Source: CAD feature listing. Evaluate the final solid. Frame: model axes, mm. Face numbers are marked on the shaded views. A direction names the side the tool comes from. Round coordinates to 2 decimals unless told otherwise and drop trailing zeros. Write each loop counter-clockwise with the first axis right and the second up, starting at its lowest first coordinate (ties: lowest second). Pieces come first, ordered by that corner, then holes. Notation, with made-up numbers: (-5.5, 10.5) -> (19.5, 10.5) arc R16 ccw to (19.5, 22.5) -> close; hole circle Ø8 at (17.5, 58). An arc over 180 degrees is marked (long way). Put each result on its own line as item: value.
```python
from build123d import *

# Parameters (mm, degrees)
F1_DEPTH    = 76.2
F2_R        = 5.08
F3_T1_DEPTH = 76.2
F3_T4_ANGLE = 106.3398594687
F3_T6_ANGLE = 106.3398594687
F4_R        = 7.7543468395
F5_DEPTH    = 0.254
F6_DEPTH    = 5.08
F7_R        = 7.6382634684
F8_DEPTH    = 5.08
F10_R       = 7.2706121331
F11_DEPTH   = 5.08
F9_R        = 7.2450103535
F12_DEPTH   = 5.08
F13_R       = 2.3168995741
F14_DEPTH   = 10.16


# Not quite as in the source:
# - a fillet or chamfer that OpenCascade refuses, or shapes differently, is made with other operations: its cross-section is extruded or revolved along the edge and cut away or added
# - the program builds the solid bodies; features that only make, move or delete a surface that nothing else refers to are left out


with BuildPart() as f1:
    # F0 (on Front) → F1 (new body)
    with BuildSketch(Plane.XZ):
        Polygon((-120.808057487, 0), (-130.5492073298, -33.2263112068), (126.3735592365, -33.2263112068), (118.6618208885, 7.3618022725), (26.1209160089, 7.3618022725), (26.1209160089, 33.3381965756), (-76.9728943706, 33.3381965756), align=None)
    extrude(amount=F1_DEPTH)

    # F2
    f2_edges = [f1.edges().sort_by_distance(p)[0] for p in [
        (-125.678632, -76.2, -16.613156),
        (-98.890476, -76.2, 16.669098),
        (-25.425989, -76.2, 33.338197),
        (26.120916, -76.2, 20.349999),
        (26.120916, 0, 20.349999),
        (26.120916, -38.1, 33.338197),
        (-98.890476, 0, 16.669098),
        (-25.425989, 0, 33.338197),
        (-125.678632, 0, -16.613156),
        (-2.087824, 0, -33.226311),
        (-120.808057, -38.1, 0),
        (-2.087824, -76.2, -33.226311),
        (72.391368, -76.2, 7.361802),
        (118.661821, -38.1, 7.361802),
        (122.51769, -76.2, -12.932254),
        (126.373559, -38.1, -33.226311),
        (122.51769, 0, -12.932254),
        (72.391368, 0, 7.361802),
    ]]
    fillet(f2_edges, radius=F2_R)

    # F3: fillet of radius 12.7 on 1 edges, made by hand

    # F3_s2 → F3_t1 (cut)
    with BuildSketch(Plane.XZ):
        with BuildLine():
            ThreePointArc((-125.7783735266, -16.9533648691), (-123.756623344, -28.1392469582), (-113.5913289929, -33.2263112068))
            Line((-113.5913289929, -33.2263112068), (-130.5492073298, -33.2263112068))
            Line((-130.5492073298, -33.2263112068), (-125.7783735266, -16.9533648691))
        make_face()
    extrude(amount=F3_T1_DEPTH, mode=Mode.SUBTRACT)

    # F3_s3 → F3_t4 (revolve, cut)
    with BuildSketch(Plane.YZ.offset(-113.5913289929)):
        with BuildLine():
            ThreePointArc((0, -28.1463112068), (-1.4878975516, -31.7384136552), (-5.08, -33.2263112068))
            Line((-5.08, -33.2263112068), (0, -33.2263112068))
            Line((0, -33.2263112068), (0, -28.1463112068))
        make_face()
    revolve(axis=Axis((-113.5913289929, 0, -20.5263112068), (0, 1, 0)), revolution_arc=F3_T4_ANGLE, mode=Mode.SUBTRACT)

    # F3_s5 → F3_t6 (revolve, cut)
    with BuildSketch(Plane(origin=(-14.5321554702, 0, -49.5680620824), x_dir=(0, 1, 0), z_dir=(0.2813343573, 0, 0.9596098058))):
        with BuildLine():
            ThreePointArc((-76.2, 110.848596585), (-74.7121024484, 114.4406990334), (-71.12, 115.928596585))
            Line((-71.12, 115.928596585), (-76.2, 115.928596585))
            Line((-76.2, 115.928596585), (-76.2, 110.848596585))
        make_face()
    revolve(axis=Axis((-113.5913289929, -76.2, -20.5263112068), (0, -1, 0)), revolution_arc=F3_T6_ANGLE, mode=Mode.SUBTRACT)

    # F4 (on face) → F5 (join)
    with BuildSketch(Plane.XZ.offset(76.2)):
        with Locations((-106.6796183586, -18.6145938933)):
            Circle(F4_R)
    extrude(amount=F5_DEPTH)

    # F6 (add): a face of the model
    f6_faces = [f1.faces().sort_by_distance(p)[0] for p in [
        (-106.6796183586, -76.454, -18.6145938933),
    ]]
    extrude(f6_faces, amount=F6_DEPTH)

    # F7 (on face) → F8 (join)
    with BuildSketch(Plane(origin=(0, 0, 0), x_dir=(-1, 0, 0), z_dir=(0, 1, 0))):
        with Locations((107.014529407, -18.2879995555)):
            Circle(F7_R)
    extrude(amount=F8_DEPTH)

    # F10 (on face) → F11 (join)
    with BuildSketch(Plane(origin=(0, 0, 0), x_dir=(-1, 0, 0), z_dir=(0, 1, 0))):
        with Locations((-98.7254753709, -20.7264013588)):
            Circle(F10_R)
    extrude(amount=F11_DEPTH)

    # F9 (on face) → F12 (join)
    with BuildSketch(Plane.XZ.offset(76.2)):
        with Locations((99.0302711725, -20.4215999693)):
            Circle(F9_R)
    extrude(amount=F12_DEPTH)

    # F13 (on face) → F14 (join)
    with BuildSketch(Plane(origin=(-44.2704434122, 0, 58.2095706289), x_dir=(0.7959568218, 0, 0.6053533991), z_dir=(-0.6053533991, 0, 0.7959568218))):
        with Locations((-89.274123311, -10.5928946286)):
            Circle(F13_R)
    extrude(amount=F14_DEPTH)


solid = f1.part
```
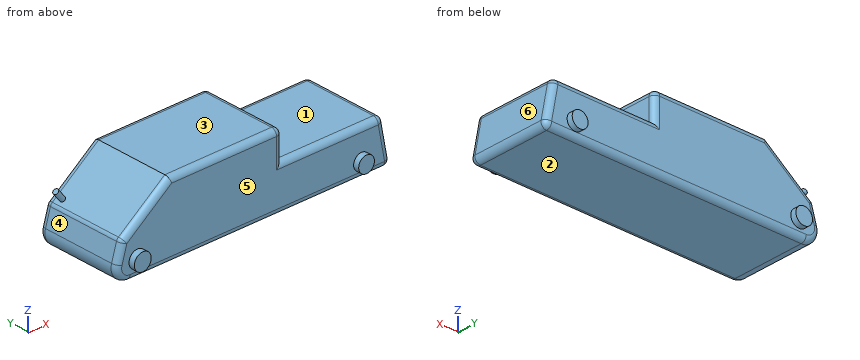
Q1. Cut plane C-C on x = -71.5. Output: boundary loops of the cut face in (y, z), and give its area (3 significant figures).
Ans:
outline: (-76.2, -28.15) arc R5.08 ccw to (-71.12, -33.23) -> (-5.08, -33.23) arc R5.08 ccw to (0, -28.15) -> (0, 28.26) arc R5.08 ccw to (-5.08, 33.34) -> (-71.12, 33.34) arc R5.08 ccw to (-76.2, 28.26) -> close
area: 5,050 mm^2
Q2. Cut plane B-B on y = -46. Output: boundary loops of the cut face in (x, z).
Ans:
outline: (-125.78, -16.95) arc R12.7 ccw to (-113.59, -33.23) -> (120.24, -33.23) arc R5.08 ccw to (125.23, -27.2) -> (119.45, 3.23) arc R5.08 ccw to (114.46, 7.36) -> (26.12, 7.36) -> (26.12, 28.26) arc R5.08 ccw to (21.04, 33.34) -> (-76.97, 33.34) -> (-119.48, 1.01) arc R5.08 ccw to (-121.28, -1.6) -> close
Q3. Draft query along X for the marked faces 3, 4, 5 and 6. Return one class per face: +X half, -X half, draft (parallel to the pull), parting line (faces both ways), or undercut.
Ans:
face 3: draft
face 4: -X half
face 5: undercut
face 6: +X half
Q4. Pin query (flat end, axial travel): pin 1 (8 mm diameter, centred on y = -6.5, z = 21, fed in from +X); pin 2 (11.5 mm diameter, centred on x = 99, z = -24, fed in from -Y); pin 3 (17 mm diameter, centred on x = 11.5, z = 3.5, fed in from +Y). Return the tip coordinate at first contact, or that it passes through.
Ans:
pin 1: stops at x = 26.12
pin 2: stops at y = -81.28
pin 3: stops at y = 0
Q5. Reachability of the marked faces 1 and 2 from +Z, -Z, +X, -X, +Y, -Y: full face, straight path, thin tool, end or side. Return the list, or none.
Ans:
face 1: +Z, +X, +Y, -Y
face 2: -Z, +X, -X, +Y, -Y
Q6. Cut plane A-A on x = 53.5. Output: boundary loops of the cut face in (y, z), and give its area (3 significant figures).
Ans:
outline: (-76.2, -28.15) arc R5.08 ccw to (-71.12, -33.23) -> (-5.08, -33.23) arc R5.08 ccw to (0, -28.15) -> (0, 2.28) arc R5.08 ccw to (-5.08, 7.36) -> (-71.12, 7.36) arc R5.08 ccw to (-76.2, 2.28) -> close
area: 3,070 mm^2
Q7. Material intervals for line 1 (Z direction, x = 91, y = -59); line 2 (Y direction, x = -50, z = 8.5); line 3 (Z direction, x = -13, y = -5), sorted ascending. Write a range as [from, to].
Ans:
line 1: z = [-33.23, 7.36]
line 2: y = [-76.2, 0]
line 3: z = [-33.23, 33.34]
